```python
from build123d import *

# Parameters (mm, degrees)
F0_R     = 17.5
F1_DEPTH = 15
F2_R     = 2


with BuildPart() as f1:
    # F0 (on Top) → F1 (new body)
    with BuildSketch(Plane.XY):
        with BuildLine():
            Line((86.187997, 25), (-68.812003, 25))
            Line((-68.812003, 25), (-68.812003, 0))
            Line((-68.812003, 0), (-68.812003, -30))
            Line((-68.812003, -30), (-58.812003, -30))
            Line((-58.812003, -30), (-58.812003, 0))
            Line((-58.812003, 0), (-48.812003, 0))
            Line((-48.812003, 0), (-48.812003, -16.553))
            Line((-48.812003, -16.553), (-40.812003, -16.553))
            Line((-40.812003, -16.553), (-40.812003, 0))
            Line((-40.812003, 0), (-30.812003, 0))
            Line((-30.812003, 0), (-23.812003, -15))
            Line((-23.812003, -15), (-16.812003, 0))
            Line((-16.812003, 0), (86.187997, 0))
            ThreePointArc((86.187997, 0), (153.879739, 12.5), (86.187997, 25))
        make_face()
        with Locations((118.879739, 12.5)):
            Circle(F0_R, mode=Mode.SUBTRACT)
    extrude(amount=F1_DEPTH)

    # F2
    f2_edges = [f1.edges().sort_by_distance(p)[0] for p in [
        (8.687997, 25, 15),
        (-68.812003, -2.5, 15),
        (-58.812003, -15, 15),
        (-48.812003, -8.2765, 15),
        (-44.812003, -16.553, 15),
        (-27.312003, -7.5, 15),
        (34.687997, 0, 15),
        (-20.312003, -7.5, 15),
        (-40.812003, -8.2765, 15),
        (-63.812003, -30, 15),
        (-53.812003, 0, 15),
        (-35.812003, 0, 15),
        (153.879739, 12.5, 15),
        (101.379739, 12.5, 15),
        (153.879739, 12.5, 0),
        (8.687997, 25, 0),
        (86.187997, 25, 7.5),
        (-68.812003, 25, 7.5),
        (34.687997, 0, 0),
        (-20.312003, -7.5, 0),
        (-27.312003, -7.5, 0),
        (-35.812003, 0, 0),
        (-40.812003, -8.2765, 0),
        (-44.812003, -16.553, 0),
        (-48.812003, -8.2765, 0),
        (-53.812003, 0, 0),
        (-58.812003, -15, 0),
        (-63.812003, -30, 0),
        (-68.812003, -2.5, 0),
    ]]
    fillet(f2_edges, radius=F2_R)


solid = f1.part
```
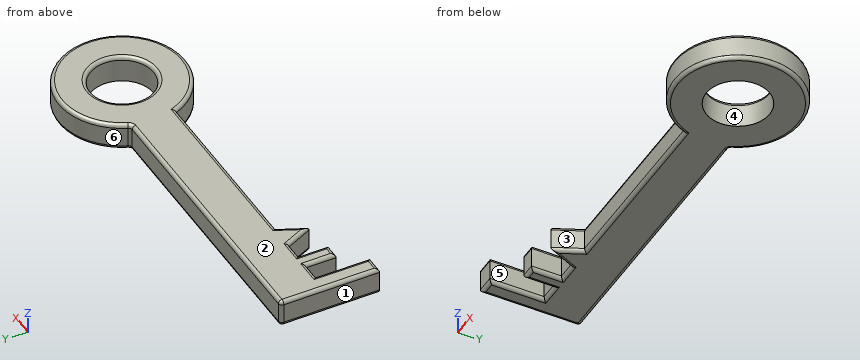
Part model, mm, in its own coordinate system. Face numbers are marked on the shaded views. A direction names the side the tool comes from. Round coordinates to 2 decimals unless told otherwise and drop trailing zeros. Write each loop counter-clockwise with the first axis right and the second up, starting at its lowest first coordinate (ties: lowest second). Pieces come first, ordered by that corner, then holes.
Item 1: Cut at A-A, the plane y = 12.5. Give the cut face in (x, z), plus the area to 3 significant figures.
Results:
outline: (-68.81, 2) arc R2 ccw to (-66.81, 0) - (101.38, 0) - (101.38, 13) arc R2 ccw to (99.38, 15) - (-66.81, 15) arc R2 ccw to (-68.81, 13) - close; (136.38, 0) - (151.88, 0) arc R2 ccw to (153.88, 2) - (153.88, 13) arc R2 ccw to (151.88, 15) - (138.38, 15) arc R2 ccw to (136.38, 13) - close
area: 2,810 mm2
Item 2: Cut at B-B, the plane z = 11. Give the cut face in (x, y).
Results:
outline: (-68.81, -30) - (-58.81, -30) - (-58.81, 0) - (-48.81, 0) - (-48.81, -16.55) - (-40.81, -16.55) - (-40.81, 0) - (-30.81, 0) - (-23.81, -15) - (-16.81, 0) - (86.19, 0) arc R35 ccw (long way) to (86.68, 26.22) arc R2 cw to (84.84, 25) - (-66.81, 25) arc R2 ccw to (-68.81, 23) - close; hole circle Ø35 at (118.88, 12.5)
Item 3: Two-plate mould, pull along X, no slides. Class the marked faces 1, 2, 3 and 4: +X half, -X half, draft (parallel to the pull), parting line (faces both ways), or undercut.
Results:
face 1: -X half
face 2: draft
face 3: undercut
face 4: undercut
Item 4: Cut at C-C, the plane x = 58. Give the cut face in (y, z), plus the area to 3 significant figures.
Results:
outline: (0, 2) arc R2 ccw to (2, 0) - (23, 0) arc R2 ccw to (25, 2) - (25, 13) arc R2 ccw to (23, 15) - (2, 15) arc R2 ccw to (0, 13) - close
area: 372 mm2
Item 5: Drop flat-ended pins along their axis: pin 1 Ø1 at (x, z) = (64.5, 6.5) entering from -Y; pin 2 Ø1.5 at (x, z) = (12.5, 2) entering from +Y; pin 3 Ø2 at (y, z) = (39.5, 8.5) entering from +X. Give the stop position or say it passes through.
Results:
pin 1: stops at y = 0
pin 2: stops at y = 25
pin 3: stops at x = 142.31
Item 6: Probe L1, parallel to X at y = 12, z = 1.75; L2, parallel to X at y = -3.5, z = 12.75; L3, parallel to X at y = -14, z = 9.75. List the from-to ranges inside material, lowest first.
Results:
L1: x = -68.8 to 101.39, 136.37 to 153.86
L2: x = -68.81 to -58.81, -48.81 to -40.81, -29.18 to -18.45, 87.75 to 111.79, 125.97 to 150.01
L3: x = -68.81 to -58.81, -48.81 to -40.81, -24.28 to -23.35, 96.02 to 141.74
Item 7: Which spindle directions (+Z, -Z, +X, -X, +Y, -Y) get a long thin tool onto all of the face, cutting with end or side? Do the marked faces 5 and 6. Say none if no direction does.
Results:
face 5: +Z, -Z, -Y
face 6: +Z, -Z
Item 8: Cut at D-D, the plane y = -12.5. Count the separate pieces of the cut face and the enclosed holes in it, plus the area to 3 significant figures.
Results:
separate pieces: 4
enclosed holes: 0
area: 1,020 mm2
